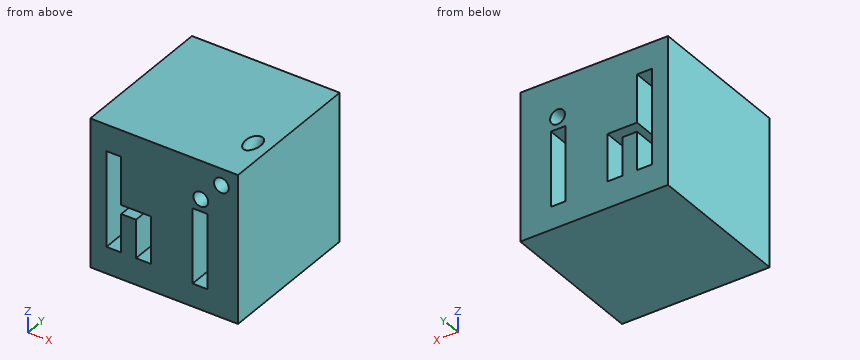
from build123d import *

# Parameters (mm, degrees)
F0_W     = 25.4
F0_H     = 25.4
F1_DEPTH = 25.4
F2_R     = 1.27
F3_DEPTH = 25.4
F4_R     = 1.27


with BuildPart() as f1:
    # F0 (on Front) → F1 (new body)
    with BuildSketch(Plane.XZ):
        with Locations((12.7, 12.7)):
            Rectangle(F0_W, F0_H)
    extrude(amount=F1_DEPTH)

    # F2 (on face) → F3 (cut)
    with BuildSketch(Plane.XZ.offset(25.4)):
        Polygon((10.399874, 12.655389), (5.319874, 12.655389), (5.319874, 20.881082), (4.538336, 20.881082), (2.779874, 20.881082), (2.779874, 4.546927), (4.538336, 4.546927), (5.319874, 4.546927), (5.319874, 11.11185), (7.859874, 11.11185), (7.859874, 4.546927), (10.399874, 4.546927), align=None)
        Polygon((20.130028, 16.778005), (17.590028, 16.768235), (17.590028, 3.921696), (20.130028, 3.921696), align=None)
        with Locations((18.996799, 18.849081)):
            Circle(F2_R)
    extrude(amount=-F3_DEPTH, mode=Mode.SUBTRACT)

    # F4 (on face) → F5 (revolve, cut)
    with BuildSketch(Plane.XZ.offset(25.4)):
        with Locations((22.5425, 22.5425)):
            Circle(F4_R)
    revolve(axis=Axis((23.53713, -25.4, 35.2425), (1, 0, 0)), mode=Mode.SUBTRACT)


solid = f1.part
Can you work these out from the model? Positions are in its coordinate system, mm. Round coordinates to 2 decimals unless told otherwise and drop trailing zeros. Order: outer loops, then holes, each group sorted by start corner. A loop starts at its lowest first (then second) coordinate and runs counter-clockwise, first axis right, second up. Notation, with made-up numbers: (20, 68.25) - (62, 68.25) arc R13 ccw to (62, 83.25) - close; hole circle Ø5 at (-25.75, -5.5). An arc over 180 degrees is marked (long way). Answer in a Markdown table with one row per item.
(1) Suppose I cut it at B-B, the plane z = 18.25. Please give me the cut outline in (x, y).
From the geometry:
| item | result |
|---|---|
| outline | (0, -25.4) - (2.78, -25.4) - (2.78, 0) - (0, 0) - close; (5.32, -25.4) - (17.88, -25.4) - (17.88, 0) - (5.32, 0) - close; (20.12, -25.4) - (25.4, -25.4) - (25.4, 0) - (20.12, 0) - close |
(2) Suppose I cut it at C-C, the plane y = -6.25. Please give me the cut outline in (x, z).
From the geometry:
| item | result |
|---|---|
| outline | (0, 0) - (25.4, 0) - (25.4, 25.4) - (0, 25.4) - close; hole (2.78, 4.55) - (5.32, 4.55) - (5.32, 11.11) - (7.86, 11.11) - (7.86, 4.55) - (10.4, 4.55) - (10.4, 12.66) - (5.32, 12.66) - (5.32, 20.88) - (2.78, 20.88) - close; hole (17.59, 3.92) - (20.13, 3.92) - (20.13, 16.78) - (17.59, 16.77) - close; hole circle Ø2.54 at (19, 18.85) |
(3) Suppose I cut it at A-A, the plane z = 5. Please give me the cut outline in (x, y).
From the geometry:
| item | result |
|---|---|
| outline | (0, -25.4) - (2.78, -25.4) - (2.78, 0) - (0, 0) - close; (5.32, -25.4) - (7.86, -25.4) - (7.86, 0) - (5.32, 0) - close; (10.4, -25.4) - (17.59, -25.4) - (17.59, 0) - (10.4, 0) - close; (20.13, -25.4) - (25.4, -25.4) - (25.4, 0) - (20.13, 0) - close |
(4) Please list where these lines run through material, in increasing order: L1, parallel to X at y = -4, z = 9; L2, parallel to X at y = -5.75, z = 12.75; L3, parallel to X at y = -12, z = 12.5. Write a range as from..to.
From the geometry:
| item | result |
|---|---|
| L1 | x = 0..2.78, 5.32..7.86, 10.4..17.59, 20.13..25.4 |
| L2 | x = 0..2.78, 5.32..17.59, 20.13..25.4 |
| L3 | x = 0..2.78, 10.4..17.59, 20.13..25.4 |
(5) Suppose I cut it at D-D, the plane y = -16.75. Count the separate pieces of the cut face and the enclosed holes in it, plus the area to 3 significant figures.
From the geometry:
| item | result |
|---|---|
| separate pieces | 1 |
| enclosed holes | 3 |
| area | 539 mm2 |
